from build123d import *

# Parameters (mm, degrees)
SKETCH1_W           = 220
SKETCH1_H           = 220
BOSS_EXTRUDE1_DEPTH = 4
SKETCH2_R           = 1.5
CUT_EXTRUDE1_DEPTH  = 8
SKETCH3_R           = 1.5
CUT_EXTRUDE2_DEPTH  = 8
CHAMFER1_SIZE       = 10
SKETCH4_R           = 1.375
CUT_EXTRUDE3_DEPTH  = 4
SKETCH5_R           = 2
CUT_EXTRUDE4_DEPTH  = 0.5
SKETCH6_W           = 42
SKETCH6_H           = 35
CUT_EXTRUDE5_DEPTH  = 0.5
SKETCH7_W           = 2.9
SKETCH7_H           = 8
CUT_EXTRUDE6_DEPTH  = 312.152695634
SKETCH9_R           = 1.5
CUT_EXTRUDE7_DEPTH  = 8
SKETCH10_R          = 1.5
CUT_EXTRUDE8_DEPTH  = 312.152695634
CUT_EXTRUDE9_DEPTH  = 46
SKETCH12_R          = 1.5
CUT_EXTRUDE11_DEPTH = 312.152695634


with BuildPart() as part:
    # Sketch1 → Boss-Extrude1 (new body)
    with BuildSketch(Plane(origin=(0, 0, 0), x_dir=(1, 0, 0), z_dir=(0, 1, 0))):
        with Locations((110, 110)):
            Rectangle(SKETCH1_W, SKETCH1_H)
    extrude(amount=BOSS_EXTRUDE1_DEPTH)

    # Sketch2 → Cut-Extrude1 (cut)
    with BuildSketch(Plane(origin=(0, 4, 0), x_dir=(1, 0, 0), z_dir=(0, 1, 0))):
        with Locations(Location((196, 4, 0), (0, 0, 270))):
            Circle(SKETCH2_R)
        with Locations(Location((158, 4, 0), (0, 0, 270))):
            Circle(SKETCH2_R)
        with Locations(Location((196, 58, 0), (0, 0, 270))):
            Circle(SKETCH2_R)
        with Locations(Location((158, 58, 0), (0, 0, 270))):
            Circle(SKETCH2_R)
    extrude(amount=-CUT_EXTRUDE1_DEPTH, mode=Mode.SUBTRACT)

    # Sketch3 → Cut-Extrude2 (cut)
    with BuildSketch(Plane(origin=(0, 4, 0), x_dir=(1, 0, 0), z_dir=(0, 1, 0))):
        with Locations(Location((62, 4, 0), (0, 0, 270))):
            Circle(SKETCH3_R)
        with Locations(Location((24, 4, 0), (0, 0, 270))):
            Circle(SKETCH3_R)
        with Locations(Location((62, 58, 0), (0, 0, 270))):
            Circle(SKETCH3_R)
        with Locations(Location((24, 58, 0), (0, 0, 270))):
            Circle(SKETCH3_R)
    extrude(amount=-CUT_EXTRUDE2_DEPTH, mode=Mode.SUBTRACT)

    # Chamfer1
    chamfer1_edges = [part.edges().sort_by_distance(p)[0] for p in [
        (0, 2, -220),
        (220, 2, -220),
        (220, 2, 0),
        (0, 2, 0),
    ]]
    chamfer(chamfer1_edges, length=CHAMFER1_SIZE)

    # Sketch4 → Cut-Extrude3 (cut)
    with BuildSketch(Plane(origin=(0, 4, 0), x_dir=(1, 0, 0), z_dir=(0, 1, 0))):
        with Locations(Location((151, 130, 0), (0, 0, 270))):
            Circle(SKETCH4_R)
        with Locations(Location((200, 130, 0), (0, 0, 270))):
            Circle(SKETCH4_R)
        with Locations(Location((151, 188, 0), (0, 0, 270))):
            Circle(SKETCH4_R)
        with Locations(Location((200, 188, 0), (0, 0, 270))):
            Circle(SKETCH4_R)
    extrude(amount=-CUT_EXTRUDE3_DEPTH, mode=Mode.SUBTRACT)

    # Sketch5 → Cut-Extrude4 (cut)
    with BuildSketch(Plane(origin=(0, 4, 0), x_dir=(1, 0, 0), z_dir=(0, 1, 0))):
        with Locations(Location((15, 205, 0), (0, 0, 270))):
            Circle(SKETCH5_R)
    extrude(amount=-CUT_EXTRUDE4_DEPTH, mode=Mode.SUBTRACT)

    # Sketch6 → Cut-Extrude5 (cut)
    with BuildSketch(Plane(origin=(0, 4, 0), x_dir=(1, 0, 0), z_dir=(0, 1, 0))):
        with Locations((177, 82.5)):
            Rectangle(SKETCH6_W, SKETCH6_H)
    extrude(amount=-CUT_EXTRUDE5_DEPTH, mode=Mode.SUBTRACT)

    # Sketch7 → Cut-Extrude6 (cut, through all)
    with BuildSketch(Plane(origin=(0, 4, 0), x_dir=(1, 0, 0), z_dir=(0, 1, 0))):
        with Locations((199.55, 82.5)):
            Rectangle(SKETCH7_W, SKETCH7_H)
        with Locations((154.45, 82.5)):
            Rectangle(SKETCH7_W, SKETCH7_H)
    extrude(amount=-CUT_EXTRUDE6_DEPTH, mode=Mode.SUBTRACT)

    # Sketch9 → Cut-Extrude7 (cut)
    with BuildSketch(Plane(origin=(0, 4, 0), x_dir=(1, 0, 0), z_dir=(0, 1, 0))):
        with Locations(Location((30, 180, 0), (0, 0, 270))):
            Circle(SKETCH9_R)
        with Locations(Location((58, 180, 0), (0, 0, 270))):
            Circle(SKETCH9_R)
        with Locations(Location((58, 131, 0), (0, 0, 270))):
            Circle(SKETCH9_R)
        with Locations(Location((30, 131, 0), (0, 0, 270))):
            Circle(SKETCH9_R)
    extrude(amount=-CUT_EXTRUDE7_DEPTH, mode=Mode.SUBTRACT)

    # Sketch10 → Cut-Extrude8 (cut, through all)
    with BuildSketch(Plane(origin=(0, 4, 0), x_dir=(1, 0, 0), z_dir=(0, 1, 0))):
        with Locations(Location((10, 210, 0), (0, 0, 270))):
            Circle(SKETCH10_R)
        with Locations(Location((10, 10, 0), (0, 0, 270))):
            Circle(SKETCH10_R)
        with Locations(Location((210, 10, 0), (0, 0, 270))):
            Circle(SKETCH10_R)
        with Locations(Location((210, 210, 0), (0, 0, 270))):
            Circle(SKETCH10_R)
    extrude(amount=-CUT_EXTRUDE8_DEPTH, mode=Mode.SUBTRACT)

    # Sketch11 → Cut-Extrude9 (cut)
    with BuildSketch(Plane(origin=(0, 4, 0), x_dir=(1, 0, 0), z_dir=(0, 1, 0))):
        with BuildLine():
            ThreePointArc((119, 194.501197137), (117.939339828, 194.061857309), (117.5, 193.001197137))
            Line((117.5, 193.001197137), (119, 193.001197137))
            Line((119, 193.001197137), (119, 194.501197137))
        make_face()
        with BuildLine():
            Line((119, 193.001197137), (117.5, 193.001197137))
            ThreePointArc((117.5, 193.001197137), (119, 191.501197137), (120.5, 193.001197137))
            ThreePointArc((120.5, 193.001197137), (120.060660172, 194.061857309), (119, 194.501197137))
            Line((119, 194.501197137), (119, 193.001197137))
        make_face()
        with BuildLine():
            ThreePointArc((101, 194.501197137), (99.939339828, 191.940536965), (102.5, 193.001197137))
            Line((102.5, 193.001197137), (101, 193.001197137))
            Line((101, 193.001197137), (101, 194.501197137))
        make_face()
        with BuildLine():
            Line((101, 193.001197137), (102.5, 193.001197137))
            ThreePointArc((102.5, 193.001197137), (102.060660172, 194.061857309), (101, 194.501197137))
            Line((101, 194.501197137), (101, 193.001197137))
        make_face()
        with BuildLine():
            ThreePointArc((102.5, 211.001197137), (99.939339828, 212.061857309), (101, 209.501197137))
            Line((101, 209.501197137), (101, 211.001197137))
            Line((101, 211.001197137), (102.5, 211.001197137))
        make_face()
        with BuildLine():
            Line((101, 211.001197137), (101, 209.501197137))
            ThreePointArc((101, 209.501197137), (102.060660172, 209.940536965), (102.5, 211.001197137))
            Line((102.5, 211.001197137), (101, 211.001197137))
        make_face()
        with BuildLine():
            ThreePointArc((117.5, 211.001197137), (117.939339828, 209.940536965), (119, 209.501197137))
            Line((119, 209.501197137), (119, 211.001197137))
            Line((119, 211.001197137), (117.5, 211.001197137))
        make_face()
        with BuildLine():
            Line((119, 211.001197137), (119, 209.501197137))
            ThreePointArc((119, 209.501197137), (120.060660172, 209.940536965), (120.5, 211.001197137))
            ThreePointArc((120.5, 211.001197137), (119, 212.501197137), (117.5, 211.001197137))
            Line((117.5, 211.001197137), (119, 211.001197137))
        make_face()
    extrude(amount=-CUT_EXTRUDE9_DEPTH, mode=Mode.SUBTRACT)

    # Sketch12 → Cut-Extrude11 (cut, through all)
    with BuildSketch(Plane(origin=(0, 4, 0), x_dir=(1, 0, 0), z_dir=(0, 1, 0))):
        with Locations(Location((141, 4, 0), (0, 0, 270))):
            Circle(SKETCH12_R)
        with Locations(Location((79, 4, 0), (0, 0, 270))):
            Circle(SKETCH12_R)
        with Locations(Location((141, 97, 0), (0, 0, 270))):
            Circle(SKETCH12_R)
        with Locations(Location((79, 97, 0), (0, 0, 270))):
            Circle(SKETCH12_R)
    extrude(amount=-CUT_EXTRUDE11_DEPTH, mode=Mode.SUBTRACT)


solid = part.part
The model under review builds one solid part; all positions refer to its coordinate system, in mm. Round coordinates to 2 decimals unless told otherwise and drop trailing zeros. Answer as a JSON object with one key per item and string values.
1. Clearance check with a flat-ended pin moving along its axis: pin 1 (2.5 mm diameter, centred on x = 24, z = -58, fed in from +Y). State where the tip first meets the part, or that it passes through.
Results found:
{"pin 1": "passes through"}
2. To check wall thickness, follow line 1 along X through (y, z) = (2.5, -58); line 2 along X through (y, z) = (2.5, -85.5); line 3 along Z through (x, y) = (141, 0.2). State the ranges of each line that lie inside material, in increasing order.
Results found:
{"line 1": "x = 0 to 22.5, 25.5 to 60.5, 63.5 to 156.5, 159.5 to 194.5, 197.5 to 220", "line 2": "x = 0 to 153, 155.9 to 198.1, 201 to 220", "line 3": "z = -220 to -98.5, -95.5 to -5.5, -2.5 to 0"}
3. The part is to be moulded in two halves that separate along X. For faces 1 (the face through (215, 2, -5)), 2 (the face through (108, 4, -112)), 3 (the face through (5, 2, -5)), 4 (the face through (177, 3.5, -83)), say which applies: pulls with the +X half, pulls with the -X half, needs draft (parallel to the pull), parting line crosses it, or undercut.
Results found:
{"face 1": "pulls with the +X half", "face 2": "needs draft", "face 3": "pulls with the -X half", "face 4": "undercut"}
